Read the model definition and answer for the solid it produces. Units are mm, in the model's axes. Face numbers are marked on the shaded views. A direction names the side the tool comes from. Give positions to 0.01 mm unless a question says otherwise; leave off trailing zeros. Loops run counter-clockwise (first coordinate to the right, second up) from the corner with the lowest first, then second, coordinate; pieces in that order, holes last. Notation, with made-up numbers: (73.25, 17) - (80.25, 17) arc R23 ccw to (80.25, 56) - close; hole circle Ø1 at (77.5, -14). An arc over 180 degrees is marked (long way). Put each result on its own line as item: value. Start each with the question number.
1. For the marked faces 1 and 2, determine the directions among +Z, -Z, +X, -X, +Y, -Y from which every point of the face is accessible in a straight line to the end or side of a thin tool.
2. A cutting plane is placed at A-A, the plane y = 0. Determine the outline of the cut face in (x, z), plus the area to 3 significant figures.
3. Given pin 1 Ø10 at (y, z) = (-11.5, 9.5) entering from -X; pin 2 Ø1.5 at (x, z) = (21.5, 10) entering from -Y; pin 3 Ø8 at (x, z) = (-38.5, -17) entering from +Y, each flat-ended and moving along its own axis, determine where each tip first touches the part or whether it passes through.
4. A cutting plane is placed at D-D, the plane z = -6.5. Determine the outline of the cut face in (x, y).
5. For a pull along Y with two mould halves and no side action, classify the marked faces 3 and 4 as released by +Y, released by -Y, zero draft, split by the parting line, or undercut.
6. A cutting plane is placed at C-C, the plane x = 0. Determine the outline of the cut face in (y, z), plus the area to 3 significant figures.
7. Consider L1, parallel to Y at x = 0, z = 13; L2, parallel to Z at x = -25.5, y = -50.5; L3, parallel to X at y = -27.5, z = -20.5. Determine where each line is inside the solid, lowest interval first. Write a range as from..to.
8. A cutting plane is placed at B-B, the plane x = 22. Determine the outline of the cut face in (y, z), plus the area to 3 significant figures.
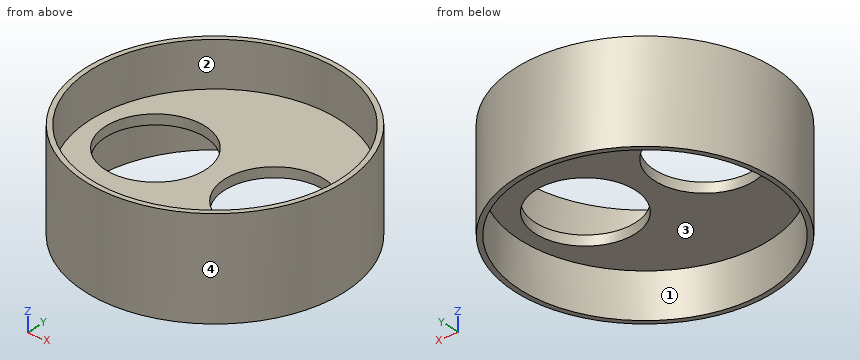
```python
from build123d import *

# Parameters (mm, degrees)
F0_R     = 66.04
F1_DEPTH = 25.4
F3_T     = -2.54
F5_D     = 50.8
F5_DEPTH = 127


with BuildPart() as f1:
    # F0 (on Top) → F1 (new body)
    with BuildSketch(Plane.XY):
        Circle(F0_R)
    extrude(amount=F1_DEPTH)

    # F3
    f3_openings = [f1.faces().sort_by_distance(p)[0] for p in [
        (0, 0, 25.4),
    ]]
    offset(amount=F3_T, openings=f3_openings)

    # F5
    with Locations(Plane(origin=(0, 0, 0), x_dir=(1, 0, 0), z_dir=(0, 0, -1))):
        with Locations((30.48, 0), (-30.48, 0)):
            Hole(F5_D / 2, depth=F5_DEPTH)

    # F6: F1 across face


with BuildPart() as f1_1:
    add(f1.part)
    add(f1.part.mirror(Plane(origin=(0, 0, 0), x_dir=(1, 0, 0), z_dir=(0, 0, -1))))


solid = f1_1.part
```
Return value:
1. face 1: -Z
1. face 2: +Z
2. outline: (-66.04, -25.4) - (-63.5, -25.4) - (-63.5, -2.54) - (-55.88, -2.54) - (-55.88, 2.54) - (-63.5, 2.54) - (-63.5, 25.4) - (-66.04, 25.4) - close; (-5.08, -2.54) - (5.08, -2.54) - (5.08, 2.54) - (-5.08, 2.54) - close; (55.88, -2.54) - (63.5, -2.54) - (63.5, -25.4) - (66.04, -25.4) - (66.04, 25.4) - (63.5, 25.4) - (63.5, 2.54) - (55.88, 2.54) - close
2. area: 387 mm2
3. pin 1: stops at x = -65.72
3. pin 2: stops at y = -62.7
3. pin 3: stops at y = 56.31
4. outline: circle Ø132.08 at (0, 0); hole circle Ø127 at (0, 0)
5. face 3: undercut
5. face 4: split by the parting line
6. outline: (-66.04, -25.4) - (-63.5, -25.4) - (-63.5, -2.54) - (63.5, -2.54) - (63.5, -25.4) - (66.04, -25.4) - (66.04, 25.4) - (63.5, 25.4) - (63.5, 2.54) - (-63.5, 2.54) - (-63.5, 25.4) - (-66.04, 25.4) - close
6. area: 903 mm2
7. L1: y = -66.04..-63.5, 63.5..66.04
7. L2: z = -2.54..2.54
7. L3: x = -60.04..-57.24, 57.24..60.04
8. outline: (-62.27, -25.4) - (-59.57, -25.4) - (-59.57, -2.54) - (-23.94, -2.54) - (-23.94, 2.54) - (-59.57, 2.54) - (-59.57, 25.4) - (-62.27, 25.4) - close; (23.94, -2.54) - (59.57, -2.54) - (59.57, -25.4) - (62.27, -25.4) - (62.27, 25.4) - (59.57, 25.4) - (59.57, 2.54) - (23.94, 2.54) - close
8. area: 636 mm2
